```python
from build123d import *

# Parameters (mm, degrees)
SKETCH1_W           = 38
SKETCH1_H           = 27
SKETCH1_H_2         = 3
SKETCH1_H_3         = 8
SKETCH1_W_2         = 8
BOSS_EXTRUDE1_DEPTH = 20
SKETCH2_R           = 4.5
BOSS_EXTRUDE2_DEPTH = 5
SKETCH3_R           = 10
BOSS_EXTRUDE3_DEPTH = 3
SKETCH4_R           = 1.5
CUT_EXTRUDE1_DEPTH  = 10
SKETCH5_R           = 1
CUT_EXTRUDE2_DEPTH  = 3
CIRPATTERN1_COUNT   = 4


with BuildPart() as part:
    # Sketch1 → Boss-Extrude1 (new body)
    with BuildSketch(Plane.XY):
        with Locations((19, 13.5)):
            Rectangle(SKETCH1_W, SKETCH1_H)
        with Locations((19, 28.5)):
            Rectangle(SKETCH1_W, SKETCH1_H_2)
        with Locations((19, 34)):
            Rectangle(SKETCH1_W, SKETCH1_H_3)
        with Locations((42, 28.5)):
            Rectangle(SKETCH1_W_2, SKETCH1_H_2)
        with Locations((-4, 28.5)):
            Rectangle(SKETCH1_W_2, SKETCH1_H_2)
    extrude(amount=BOSS_EXTRUDE1_DEPTH)

    # Sketch2 → Boss-Extrude2 (add)
    with BuildSketch(Plane(origin=(0, 38, 0), x_dir=(1, 0, 0), z_dir=(0, 1, 0))):
        with Locations((30.956279898, -10)):
            Circle(SKETCH2_R)
    extrude(amount=BOSS_EXTRUDE2_DEPTH)

    # Sketch3 → Boss-Extrude3 (add)
    with BuildSketch(Plane(origin=(0, 43, 0), x_dir=(1, 0, 0), z_dir=(0, 1, 0))):
        with Locations((30.956279898, -10)):
            Circle(SKETCH3_R)
    extrude(amount=BOSS_EXTRUDE3_DEPTH)

    # Sketch4 → Cut-Extrude1 (cut)
    with BuildSketch(Plane(origin=(0, 30, 0), x_dir=(1, 0, 0), z_dir=(0, 1, 0))):
        with Locations((42.456279898, -14.5)):
            Circle(SKETCH4_R)
        with Locations((42.456279898, -5.5)):
            Circle(SKETCH4_R)
        with Locations((-4.543720102, -14.5)):
            Circle(SKETCH4_R)
        with Locations((-4.543720102, -5.5)):
            Circle(SKETCH4_R)
    extrude(amount=-CUT_EXTRUDE1_DEPTH, mode=Mode.SUBTRACT)

    # Sketch5 → Cut-Extrude2 (cut)
    with BuildSketch(Plane(origin=(0, 46, 0), x_dir=(1, 0, 0), z_dir=(0, 1, 0))):
        with Locations((30.956279898, -4)):
            Circle(SKETCH5_R)
        with Locations((27.956279898, -4)):
            Circle(SKETCH5_R)
        with Locations((33.956279898, -4)):
            Circle(SKETCH5_R)
    cut_extrude2 = extrude(amount=-CUT_EXTRUDE2_DEPTH, mode=Mode.SUBTRACT)

    # CirPattern1: Cut-Extrude2 ×4 about axis
    cirpattern1_axis = Axis((30.956279898, 0, 10), (0, 1, 0))
    for i in range(1, CIRPATTERN1_COUNT):
        add(cut_extrude2.rotate(cirpattern1_axis, i * 360 / CIRPATTERN1_COUNT), mode=Mode.SUBTRACT)


solid = part.part
```
Input: part model. Units: mm. Frame: model coordinates. A direction names the side the tool comes from. Round coordinates to 2 decimals unless told otherwise and drop trailing zeros. Write each loop counter-clockwise with the first axis right and the second up, starting at its lowest first coordinate (ties: lowest second). Pieces come first, ordered by that corner, then holes. Notation, with made-up numbers: (45.25, -2.75) -> (92.25, -2.75) arc R15 ccw to (92.25, 7.25) -> close; hole circle Ø5 at (85.25, 5). An arc over 180 degrees is marked (long way). Answer as CSV lines item,"result".
1. Section C-C (x = 6.5). Return the cut outline in (y, z), plus the area to 3 significant figures.
Geometry says:
outline,"(0, 0) -> (38, 0) -> (38, 20) -> (0, 20) -> close"
area,"760 mm^2"
2. Contact query for flat-ended pins moving along their axis: P1, Ø10, axis at y = 19.5, z = 6, coming from the +X side; P2, Ø10, axis at y = 12.5, z = 6.5, coming from the -X side; P3, Ø1.6, axis at x = 24.96, z = 10, coming from the +Y side. Output: stop coordinate, or through.
Geometry says:
P1,"stops at x = 38"
P2,"stops at x = 0"
P3,"stops at y = 38"
3. Mould query, pull axis Y, two halves, no side actions, for faces 1 (the flat face through (-4, 27, 10)), 2 (the flat face through (19, 19, 20)), 3 (the cylindrical face through (35.25, 40.47, 8.65)). Classes: +Y half, -Y half, draft (parallel to the pull), parting line (faces both ways), or undercut.
Geometry says:
face 1,"-Y half"
face 2,"draft"
face 3,"undercut"
4. Section B-B (z = 18). Return the cut outline in (x, y), plus the area to 3 significant figures.
Geometry says:
outline,"(-8, 27) -> (0, 27) -> (0, 0) -> (38, 0) -> (38, 27) -> (46, 27) -> (46, 30) -> (38, 30) -> (38, 38) -> (0, 38) -> (0, 30) -> (-8, 30) -> close; (24.96, 43) -> (36.96, 43) -> (36.96, 46) -> (24.96, 46) -> close"
area,"1,530 mm^2"
5. Reachability of faces 4 (the flat face through (38, 13, 10)), 5 (the cylindrical face through (34.91, 44.52, 3.7)), 6 (the flat face through (42, 30, 10)), 7 (the flat face through (0, 14, 10)), 8 (the cylindrical face through (41.266, 28.521, 15.413)) from +Z, -Z, +X, -X, +Y, -Y: full face, straight path, thin tool, end or side. Return the list, or none.
Geometry says:
face 4,"+Z, -Z, +X, -Y"
face 5,"+Y"
face 6,"+Z, -Z, +X"
face 7,"+Z, -Z, -X, -Y"
face 8,"+Y, -Y"
6. Section A-A (z = 10). Return the cut outline in (x, y).
Geometry says:
outline,"(-8, 27) -> (0, 27) -> (0, 0) -> (38, 0) -> (38, 27) -> (46, 27) -> (46, 30) -> (38, 30) -> (38, 38) -> (35.46, 38) -> (35.46, 43) -> (35.96, 43) -> (35.96, 46) -> (25.96, 46) -> (25.96, 43) -> (26.46, 43) -> (26.46, 38) -> (0, 38) -> (0, 30) -> (-8, 30) -> close; (20.96, 43) -> (23.96, 43) -> (23.96, 46) -> (20.96, 46) -> close; (37.96, 43) -> (40.96, 43) -> (40.96, 46) -> (37.96, 46) -> close"
7. Ray query, L1, parallel to X at y = 28.5, z = 14.5; L2, parallel to X at y = 44.8, z = 7; L3, parallel to Y at x = 39, z = 13. Return the intervals inside material, ascending. Write a range as [from, to].
Geometry says:
L1,"x = [-8, -6.04], [-3.04, 40.96], [43.96, 46]"
L2,"x = [21.42, 23.96], [25.96, 35.96], [37.96, 40.5]"
L3,"y = [27, 30], [43, 46]"
